from build123d import *

# Parameters (mm, degrees)
F1_DEPTH = 50
F2_DEPTH = 12.5
F3_DEPTH = 5
F5_R     = 5


with BuildPart() as f1:
    # F0 (on Front) → F1 (new body, symmetric)
    with BuildSketch(Plane.XZ):
        Polygon((-31.3122831285, 15), (-50, 15), (-50, -15), (50, -15), (50, 15), (40, 15), align=None)
    extrude(amount=F1_DEPTH, both=True)

    # F0 (on Front) → F2 (join, symmetric)
    with BuildSketch(Plane.XZ):
        with BuildLine():
            Line((40, 44.0615866161), (40, 15))
            Line((40, 15), (50, 15))
            Line((50, 15), (50, 44.0615866161))
            ThreePointArc((50, 44.0615866161), (53.2037871047, 51.7962128953), (60.9384133839, 55))
            Line((60.9384133839, 55), (75, 55))
            Line((75, 55), (75, 64.9994979734))
            add(Edge.make_bspline(
                [(75, 64.9994979734), (67.590366239, 64.98362656), (60.6448722372, 64.59168303), (54.1236525971, 63.8599751984)],
                knots=[0.3245366314, 0.3245366314, 0.3245366314, 0.3245366314, 15.7199359846, 15.7199359846, 15.7199359846, 15.7199359846], degree=3))
            ThreePointArc((54.1236525971, 63.8599751984), (43.8927770875, 56.2214977294), (40, 44.0615866161))
        make_face()
        with BuildLine():
            add(Edge.make_bspline(
                [(75.469206692, 65), (75.3125979622, 65), (75.156195856, 64.9998325444), (75, 64.9994979734)],
                knots=[0, 0, 0, 0, 0.3245366314, 0.3245366314, 0.3245366314, 0.3245366314], degree=3))
            Line((75, 64.9994979734), (75, 55))
            Line((75, 55), (90, 55))
            Line((90, 55), (90, 65))
            Line((90, 65), (75.469206692, 65))
        make_face()
    extrude(amount=F2_DEPTH, both=True)

    # F0 (on Front) → F3 (join, symmetric)
    with BuildSketch(Plane.XZ):
        with BuildLine():
            add(Edge.make_bspline(
                [(54.1236525971, 63.8599751984), (10.8386087283, 59.0032141413), (-13.7540441275, 39.1773487702), (-31.3122831285, 15)],
                knots=[15.7199359846, 15.7199359846, 15.7199359846, 15.7199359846, 117.9079580362, 117.9079580362, 117.9079580362, 117.9079580362], degree=3))
            Line((-31.3122831285, 15), (40, 15))
            Line((40, 15), (40, 44.0615866161))
            ThreePointArc((40, 44.0615866161), (43.8927770875, 56.2214977294), (54.1236525971, 63.8599751984))
        make_face()
    extrude(amount=F3_DEPTH, both=True)

    # F0 (on Front) → F4 (revolve)
    with BuildSketch(Plane.XZ):
        Polygon((90, 65), (90, 55), (90, 50), (105, 50), (105, 70), (90, 70), align=None)
    revolve(axis=Axis((90, 0, 60), (0, 0, -1)))

    # F5
    f5_edges = [f1.edges().sort_by_distance(p)[0] for p in [
        (50, -50, 0),
        (-50, -50, 0),
        (50, 50, 0),
        (-50, 50, 0),
        (0, 50, 15),
        (-50, 0, 15),
        (0, -50, 15),
        (50, -31.25, 15),
        (50, 31.25, 15),
    ]]
    fillet(f5_edges, radius=F5_R)


solid = f1.part
Read the model definition and answer for the solid it produces. Units are mm, in the model's axes. A direction names the side the tool comes from. Round coordinates to 2 decimals unless told otherwise and drop trailing zeros. Loops run counter-clockwise (first coordinate to the right, second up) from the corner with the lowest first, then second, coordinate; pieces in that order, holes last.
Q1. Section D-D on x = 90 is taken. Write down the section's boundary in (y, z), and give its area (3 significant figures).
Q2. Determine the mould class of faces 5 (the face through (53.12, -0.18, 51.71)), 6 (the face through (49, -29, 13)), 7 (the face through (-50, -1, -2)), 8 (the face through (77, -10, 65)) for opening direction X: released by +X, released by -X, zero draft, split by the parting line, or undercut.
Q3. Which of the six approach directions +Z, -Z, +X, -X, +Y, -Y give full straight-line access (tool end or side, diameter ignored) to faces 1 (the face through (40, -9, 30)), 2 (the face through (44, 8.7, 56.37)), 3 (the face through (-48, 1, 14)), 4 (the face through (50, -1, 8))?
Q4. Each of these flat-tipped pins is pushed along its axis until it touches: pin 1 (12 mm diameter, centred on x = 52.5, z = 15.5, fed in from -Y); pin 2 (8 mm diameter, centred on y = 9.5, z = 25, fed in from -X); pin 3 (21 mm diameter, centred on x = 60, z = 28.5, fed in from -Y); pin 4 (3 mm diameter, centred on x = 77.5, y = 9.5, fed in from +Z). Where does it stop, or does it pass through?
Q5. Section A-A on z = -7.5 is taken. Write down the section's boundary in (x, y).
Q6. Section B-B on y = 36.5 is taken. Write down the section's boundary in (x, z).
Q7. Consider probe 1 along Z at (x, y) = (-10.5, 9); probe 2 along Y at (x, z) = (25, 50.5); probe 3 along Y at (x, z) = (56, 62.5). Determine where each line is inside the solid, lowest interval first.
Output:
1. outline: (-15, 50) - (15, 50) - (15, 70) - (-15, 70) - close
1. area: 600 mm2
2. face 5: undercut
2. face 6: released by +X
2. face 7: released by -X
2. face 8: zero draft
3. face 1: +Z, -X, -Y
3. face 2: +Z, -X, +Y
3. face 3: +Z, -X, +Y, -Y
3. face 4: -Z, +X, +Y, -Y
4. pin 1: stops at y = -48.76
4. pin 2: stops at x = 40
4. pin 3: stops at y = -12.5
4. pin 4: stops at z = 70
5. outline: (-50, -45) arc R5 ccw to (-45, -50) - (45, -50) arc R5 ccw to (50, -45) - (50, 45) arc R5 ccw to (45, 50) - (-45, 50) arc R5 ccw to (-50, 45) - close
6. outline: (-50, -15) - (50, -15) - (50, 10) arc R5 ccw to (45, 15) - (-45, 15) arc R5 ccw to (-50, 10) - close
7. probe 1: z = -15 to 15
7. probe 2: y = -5 to 5
7. probe 3: y = -12.5 to 12.5
